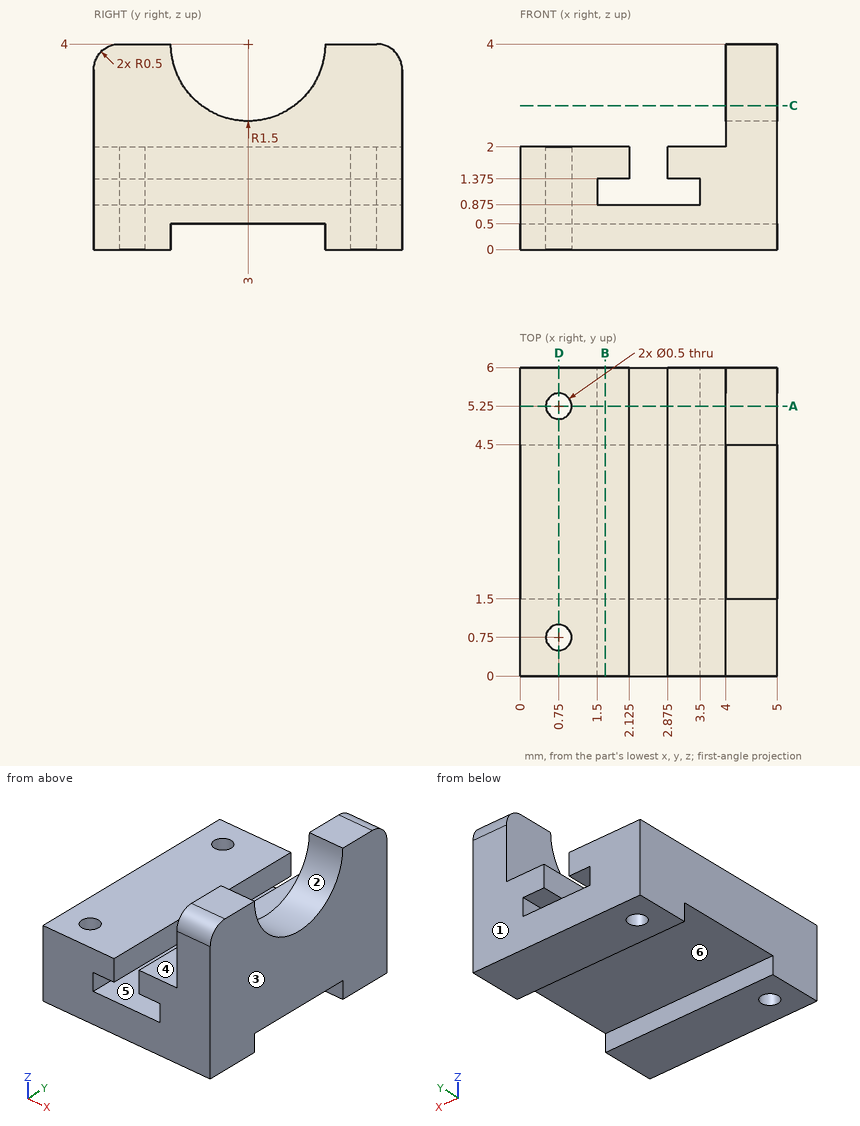
Geometry: see drawing. Coordinates: mm, zero at the bounding-box minimum. A direction names the side the tool comes from. Give positions to 0.01 mm unless a question says otherwise; leave off trailing zeros. Order: outer loops, then holes, each group sorted by start corner. A loop starts at its lowest first (then second) coordinate and runs counter-clockwise, first axis right, second up. Notation, with made-up numbers: (7, 64.5) -> (60, 64.5) arc R15 ccw to (60, 68.5) -> close; hole circle Ø8 at (59.5, 44.25). An arc over 180 degrees is marked (long way). Write each question's results on one line, items separated by ' | '. Start each with the question number.
1) Draft query along Y for the marked faces 1, 2 and 3. Return one class per face: pulls with the +Y half, pulls with the -Y half, needs draft (parallel to the pull), parting line crosses it, or undercut.
2) Line query: line 1 (Y direction, x = 0.75, z = 1.1); line 2 (Y direction, x = 0.75, z = 0.4); line 3 (X direction, y = 1.45, z = 1.65) (3 decimals). Output: solid intervals per line, ascending. Write a range as from..to.
3) Section A-A (y = 5.25). Return loops of the section in (x, z) (3 decimals), then the cut area to 3 significant figures.
4) Section D-D (x = 0.75). Return loops of the section in (y, z), then the cut area to 3 significant figures.
5) Section B-B (x = 1.65). Return loops of the section in (y, z) (3 decimals).
6) First-contact query: pin 1 (0.6 mm diameter, centred on x = 2.5, y = 4, fed in from +Z) (3 decimals); pin 2 (1.7 mm diameter, centred on x = 1.5, y = 4, fed in from +Z); pin 3 (2.5 mm diameter, centred on x = 3, y = 3, fed in from -Z). Flat tips, straight axial feed; report the tip coordinate or a pass-through.
7) Set-up query: the marked faces 4, 5 and 6. Return all of +Z, -Z, +X, -X, +Y, -Y with unobstructed straight access to the full face (end or side cutting, diameter ignored); none if empty.
8) Section C-C (z = 2.8). Return loops of the section in (x, y), then the cut area to 3 significant figures.
Calculated:
1) face 1: pulls with the +Y half | face 2: undercut | face 3: needs draft
2) line 1: 0..0.5, 1..5, 5.5..6 | line 2: 0..0.5, 1..1.5, 4.5..5, 5.5..6 | line 3: 0..2.125, 2.875..5
3) outline: (0, 0) -> (0.5, 0) -> (0.5, 2) -> (0, 2) -> close; (1, 0) -> (5, 0) -> (5, 4) -> (4, 4) -> (4, 2) -> (2.875, 2) -> (2.875, 1.375) -> (3.5, 1.375) -> (3.5, 0.875) -> (1.5, 0.875) -> (1.5, 1.375) -> (2.125, 1.375) -> (2.125, 2) -> (1, 2) -> close | area: 9.53 mm2
4) outline: (0, 0) -> (0.5, 0) -> (0.5, 2) -> (0, 2) -> close; (1, 0) -> (1.5, 0) -> (1.5, 0.5) -> (4.5, 0.5) -> (4.5, 0) -> (5, 0) -> (5, 2) -> (1, 2) -> close; (5.5, 0) -> (6, 0) -> (6, 2) -> (5.5, 2) -> close | area: 8.50 mm2
5) outline: (0, 0) -> (1.5, 0) -> (1.5, 0.5) -> (4.5, 0.5) -> (4.5, 0) -> (6, 0) -> (6, 0.875) -> (0, 0.875) -> close; (0, 1.375) -> (6, 1.375) -> (6, 2) -> (0, 2) -> close
6) pin 1: z = 0.875 | pin 2: z = 2 | pin 3: z = 0.5
7) face 4: +Z, -X, +Y, -Y | face 5: +Y, -Y | face 6: -Z, +X, -X
8) outline: (4, 0) -> (5, 0) -> (5, 2.1) -> (4, 2.1) -> close; (4, 3.9) -> (5, 3.9) -> (5, 6) -> (4, 6) -> close | area: 4.20 mm2
